from build123d import *

# Parameters (mm, degrees)
SKETCH1_W                  = 16
SKETCH1_H                  = 15
BOSS_EXTRUDE1_DEPTH        = 2
SKETCH4_W                  = 2
SKETCH4_H                  = 15
BOSS_EXTRUDE4_DEPTH        = 28
F_3_2_3_2_DIAMETER_SLOT1_D = 3.2
M4_CLEARANCE_SLOT1_D       = 4.5


with BuildPart() as part:
    # Sketch1 → Boss-Extrude1 (new body)
    with BuildSketch(Plane(origin=(0, 0, 0), x_dir=(1, 0, 0), z_dir=(0, 1, 0))):
        with Locations((4.176470588, 2.588235294)):
            Rectangle(SKETCH1_W, SKETCH1_H)
    extrude(amount=BOSS_EXTRUDE1_DEPTH)

    # Sketch4 → Boss-Extrude4 (add)
    with BuildSketch(Plane(origin=(0, 2, 0), x_dir=(1, 0, 0), z_dir=(0, 1, 0))):
        with Locations((-2.823529412, 2.588235294)):
            Rectangle(SKETCH4_W, SKETCH4_H)
    extrude(amount=BOSS_EXTRUDE4_DEPTH)

    # Ø3.2 (3.2) Diameter Slot1 (through all)
    with Locations(Plane(origin=(0, 2, 0), x_dir=(1, 0, 0), z_dir=(0, 1, 0))):
        with Locations((6.972823148, 6.088235294), (6.972823148, -0.911764706)):
            Hole(F_3_2_3_2_DIAMETER_SLOT1_D / 2)

    # M4 Clearance Slot1 (through all)
    with Locations(Plane(origin=(-1.823529412, 0, 0), x_dir=(0, 0, -1), z_dir=(1, 0, 0))):
        with Locations((2.588235294, 18.5)):
            Hole(M4_CLEARANCE_SLOT1_D / 2)


solid = part.part
CAD build for the part. Positions are in the model's coordinates, mm. A direction names the side the tool comes from. Give positions to 0.01 mm unless a question says otherwise; leave off trailing zeros. Order: outer loops, then holes, each group sorted by start corner. A loop starts at its lowest first (then second) coordinate and runs counter-clockwise, first axis right, second up. Notation, with made-up numbers: (64, 3) - (106, 3) arc R15 ccw to (106, 12) - close; hole circle Ø2 at (19.5, 33). An arc over 180 degrees is marked (long way). Write each question's results on one line, items separated by ' | '.
1. Saw through at A-A on y = 18.5. List the corners of the cut face in (x, z), and give its area (3 significant figures).
Calculated:
outline: (-3.82, -10.09) - (-1.82, -10.09) - (-1.82, -4.84) - (-3.82, -4.84) - close; (-3.82, -0.34) - (-1.82, -0.34) - (-1.82, 4.91) - (-3.82, 4.91) - close | area: 21.0 mm2
2. Probe L1, parallel to Y at x = 1.75, z = 0.5; L2, parallel to X at y = 9.5, z = 4. List the from-to ranges inside material, lowest first. Write a range as from..to.
Calculated:
L1: y = 0..2 | L2: x = -3.82..-1.82
3. Saw through at D-D on z = -5.5. List the corners of the cut face in (x, y).
Calculated:
outline: (-3.82, 0) - (5.48, 0) - (5.48, 2) - (-1.82, 2) - (-1.82, 30) - (-3.82, 30) - close; (8.46, 0) - (12.18, 0) - (12.18, 2) - (8.46, 2) - close
4. Saw through at B-B on z = -3.75. List the corners of the cut face in (x, y), and give its area (3 significant figures).
Calculated:
outline: (-3.82, 0) - (12.18, 0) - (12.18, 2) - (-1.82, 2) - (-1.82, 16.57) - (-3.82, 16.57) - close; (-3.82, 20.43) - (-1.82, 20.43) - (-1.82, 30) - (-3.82, 30) - close | area: 80.3 mm2
5. Pull direction Z, two halves, no side cores. Call faces 1 (the face through (-3, 30, -3)), 2 (the face through (-2.838, 16.304, -3.076)), 3 (the face through (-2, 10, 4.912)): released by +Z, released by -Z, zero draft, split by the parting line, or undercut.
Calculated:
face 1: zero draft | face 2: undercut | face 3: released by +Z
6. 3-axis set-ups, long thin cutter, end or side, ignore diameter. For faces 4 (the face through (12.176, 1, -2)), 5 (the face through (-1.824, 16, -2)): which of +Z, -Z, +X, -X, +Y, -Y reach the whole face in a straight line?
Calculated:
face 4: +Z, -Z, +X, +Y, -Y | face 5: +Z, -Z, +X, +Y
7. Saw through at C-C on x = 4.5. List the corners of the cut face in (y, z), and give its area (3 significant figures).
Calculated:
outline: (0, -10.09) - (2, -10.09) - (2, 4.91) - (0, 4.91) - close | area: 30.0 mm2
8. Pin check, flat tips, straight feed: pin 1 (4 mm diameter, centred on y = 24, z = -3.5, fed in from +X); pin 2 (4 mm diameter, centred on x = 2, z = 1, fed in from +Y); pin 3 (5 mm diameter, centred on x = 6.97, z = -6.09, fed in from -Y). Stop position of each tip, or through.
Calculated:
pin 1: stops at x = -1.82 | pin 2: stops at y = 2 | pin 3: stops at y = 0
